Study the drawing (mm; zero at the part's minimum x, y, z) and answer. A direction names the side the tool comes from. Coordinates: 2 decimals unless noted, no trailing zeros. Loops run counter-clockwise (first coordinate to the right, second up) from the corner with the lowest first, then second, coordinate; pieces in that order, holes last. Notation, with made-up numbers: (73, -34.5) - (111, -34.5) arc R24 ccw to (111, -5.5) - close; hole circle Ø2 at (44, 47.5). An arc over 180 degrees is marked (long way). Put each result on its own line as item: value.
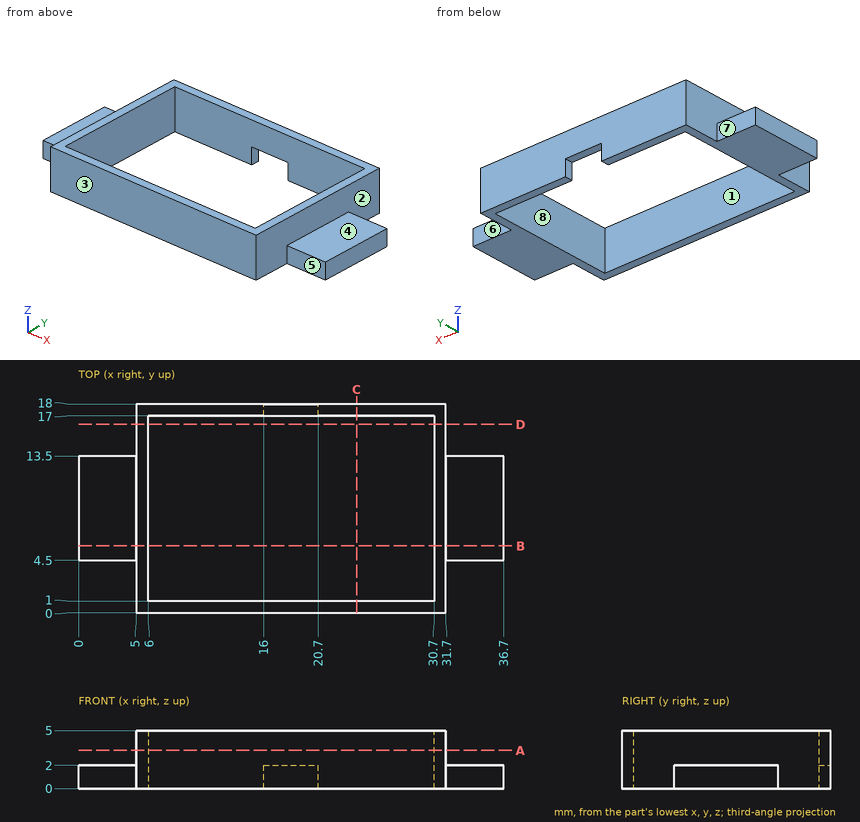
1) For a pull along Y with two mould halves and no side action, classify the marked faces 1, 2 and 3 as pulls with the +Y half, pulls with the -Y half, needs draft (parallel to the pull), parting line crosses it, or undercut.
Found:
face 1: undercut
face 2: needs draft
face 3: pulls with the -Y half
2) The part is cut by section C-C (x = 24). Give the vertices of the cut face in (y, z), and give its area (3 significant figures).
Found:
outline: (0, 0) - (1, 0) - (1, 5) - (0, 5) - close; (17, 0) - (18, 0) - (18, 5) - (17, 5) - close
area: 10.0 mm^2
3) The part is cut by section A-A (z = 3.3). Give the vertices of the cut face in (x, y), and give its area (3 significant figures).
Found:
outline: (5, 0) - (31.7, 0) - (31.7, 18) - (5, 18) - close; hole (6, 1) - (30.7, 1) - (30.7, 17) - (6, 17) - close
area: 85.4 mm^2
4) The part is cut by section B-B (y = 5.75). Give the vertices of the cut face in (x, z).
Found:
outline: (0, 0) - (6, 0) - (6, 5) - (5, 5) - (5, 2) - (0, 2) - close; (30.7, 0) - (36.7, 0) - (36.7, 2) - (31.7, 2) - (31.7, 5) - (30.7, 5) - close
5) The part is cut by section D-D (y = 16.25). Give the vertices of the cut face in (x, z).
Found:
outline: (5, 0) - (6, 0) - (6, 5) - (5, 5) - close; (30.7, 0) - (31.7, 0) - (31.7, 5) - (30.7, 5) - close
6) Straight lines are drawn through the part: L1, parallel to X at y = 10.25, z = 1.9; L2, parallel to Y at x = 25, z = 3.6; L3, parallel to X at y = 2.25, z = 1. For each, find the intervals that lie inside material, in ascending order. Write a range as [from, to].
Found:
L1: x = [0, 6], [30.7, 36.7]
L2: y = [0, 1], [17, 18]
L3: x = [5, 6], [30.7, 31.7]
7) Each of these flat-tipped pins is pushed along its axis until it touches: pin 1 (1.5 mm diameter, centred on y = 11, z = 2.5, fed in from +X); pin 2 (1.1 mm diameter, centred on x = 19, y = 17.5, fed in from -Z); pin 3 (0.6 mm diameter, centred on x = 3, z = 0.5, fed in from +Y); pin 4 (0.6 mm diameter, centred on x = 35.5, z = 0.5, fed in from -Y). Where does it stop, or does it pass through?
Found:
pin 1: stops at x = 36.7
pin 2: stops at z = 2
pin 3: stops at y = 13.5
pin 4: stops at y = 4.5
8) For the marked faces 4, 5, 6, 7 and 8, determine the directions among +Z, -Z, +X, -X, +Y, -Y from which every point of the face is accessible in a straight line to the end or side of a thin tool.
Found:
face 4: +Z, +X, +Y, -Y
face 5: +Z, -Z, +X, -Y
face 6: +Z, -Z, +X, +Y
face 7: +Z, -Z, -X, +Y
face 8: +Z, -Z
